The listing builds one solid part. Answer for the finished solid, in the listing's coordinates (mm). A direction names the side the tool comes from. Coordinates: 2 decimals unless noted, no trailing zeros. Write each loop counter-clockwise with the first axis right and the second up, starting at its lowest first coordinate (ties: lowest second). Pieces come first, ordered by that corner, then holes.
(1) For a pull along Z with two mould halves and no side action, classify faces 1 (the cylindrical face through (-1.669, 1.972, -23.347)), 2 (the cylindrical face through (12.61, 1.97, 8.82)), 3 (the cylindrical face through (6.76, 1.97, 10.83)), 4 (the cylindrical face through (6.792, 1.972, 6.686)) as +Z half, -Z half, draft (parallel to the pull), parting line (faces both ways), or undercut.
(2) The part is cut by section A-A on x = -2.5. Determine the outline of the cut face in (y, z), plus the area to 3 significant figures.
(3) The part is cut by section B-B on z = -19.5. Determine the outline of the cut face in (x, y).
(4) The part is cut by section D-D on x = 7. Determine the outline of the cut face in (y, z).
(5) Which of the six approach directions +Z, -Z, +X, -X, +Y, -Y give full straight-line access (tool end or side, diameter ignored) to faces 5 (the flat face through (4.24, 1.97, -0.21)), 6 (the flat face through (-3.874, 1.972, 19.331)), 7 (the cylindrical face through (0.325, 1.972, 17.289)), 8 (the flat face through (7.2, 2, 2.8)), 9 (the flat face through (0, 0, 5))?
(6) Straight lines are drawn through the part: line 1 (Z direction, x = 6.5, y = 2.9); line 2 (Z direction, x = -2.25, y = 3.1); line 3 (X direction, y = 3, z = -6). For each, find the intervals that lie inside material, in ascending order.
(7) Given P1, Ø2, axis at y = 2, z = -13.5, coming from the -X side; P2, Ø1.5, axis at y = 1.5, z = 2, coming from the +X side, each flat-ended and moving along its own axis, determine where each tip first touches the part or whether it passes through.
(8) The part is cut by section C-C on y = 0.75. Give the number of separate pieces and of enclosed holes in the cut face, plus the area to 3 significant figures.
from build123d import *

# Parameters (mm, degrees)
CROQUIS1_R              = 1.500000449
CROQUIS1_R_2            = 1.500000067
SALIENTE_EXTRUIR1_DEPTH = 4


with BuildPart() as part:
    # Croquis1 → Saliente-Extruir1 (new body)
    with BuildSketch(Plane(origin=(0, 0, 0), x_dir=(1, 0, 0), z_dir=(0, 1, 0))):
        with BuildLine():
            Line((7.803034841, -10.666075678), (9.826177161, -11.05442464))
            ThreePointArc((9.826177161, -11.05442464), (12.611497219, -8.758438746), (9.837059372, -6.449314739))
            Line((9.837059372, -6.449314739), (7.783190104, -6.83350636))
            ThreePointArc((7.783190104, -6.83350636), (6.778877321, -6.678958506), (6.091539896, -5.930562574))
            Line((6.091539896, -5.930562574), (5.8088579, -5.271694401))
            ThreePointArc((5.8088579, -5.271694401), (5.746747512, -4.205872048), (6.380859817, -3.346956119))
            Line((6.380859817, -3.346956119), (8.045875641, -2.237519038))
            ThreePointArc((8.045875641, -2.237519038), (8.404769789, 1.386225416), (4.781168268, 1.025891001))
            Line((4.781168268, 1.025891001), (3.675334506, -0.635147383))
            ThreePointArc((3.675334506, -0.635147383), (2.774259756, -1.283481634), (1.669267023, -1.177349334))
            Line((1.669267023, -1.177349334), (1.3673448, -1.048666977))
            Line((1.3673448, -1.048666977), (1.3673448, 20.24263647))
            ThreePointArc((1.3673448, 20.24263647), (-1.737654981, 23.347636251), (-4.842654762, 20.24263647))
            Line((-4.842654762, 20.24263647), (-4.842654762, 0.571999527))
            ThreePointArc((-4.842654762, 0.571999527), (-11.591302814, -9.338185795), (-3.698262021, -18.363479735))
            Line((-3.698262021, -18.363479735), (-4.053895188, -20.326281833))
            ThreePointArc((-4.053895188, -20.326281833), (-1.716098294, -23.09980655), (0.570509604, -20.283930489))
            Line((0.570509604, -20.283930489), (0.177742699, -18.321752082))
            ThreePointArc((0.177742699, -18.321752082), (0.331674177, -17.275555509), (1.114410942, -16.564538403))
            Line((1.114410942, -16.564538403), (1.762991063, -16.295067607))
            ThreePointArc((1.762991063, -16.295067607), (2.82080022, -16.242583246), (3.671047948, -16.874084331))
            Line((3.671047948, -16.874084331), (4.780498307, -18.539119038))
            ThreePointArc((4.780498307, -18.539119038), (8.406487962, -18.895762792), (8.038611241, -15.270895558))
            Line((8.038611241, -15.270895558), (6.389450023, -14.179385265))
            ThreePointArc((6.389450023, -14.179385265), (5.741374186, -13.307833185), (5.800109712, -12.223326174))
            Line((5.800109712, -12.223326174), (6.067644855, -11.592044841))
            ThreePointArc((6.067644855, -11.592044841), (6.771618308, -10.822224208), (7.803034841, -10.666075678))
        make_face()
        with Locations((-1.73765539, 20.242635654)):
            Circle(CROQUIS1_R, mode=Mode.SUBTRACT)
        with Locations((-1.737655616, -8.757364808)):
            Circle(CROQUIS1_R_2, mode=Mode.SUBTRACT)
    extrude(amount=SALIENTE_EXTRUIR1_DEPTH)


solid = part.part
Model answer:
1. face 1: -Z half
1. face 2: parting line
1. face 3: undercut
1. face 4: undercut
2. outline: (0, -23.25) - (4, -23.25) - (4, -21.53) - (0, -21.53) - close; (0, -18.95) - (4, -18.95) - (4, 7.47) - (0, 7.47) - close; (0, 10.05) - (4, 10.05) - (4, 22.97) - (0, 22.97) - close
2. area: 164 mm2
3. outline: (-4.84, 0) - (-3.04, 0) - (-3.04, 4) - (-4.84, 4) - close; (-0.43, 0) - (1.37, 0) - (1.37, 4) - (-0.43, 4) - close
4. outline: (0, -2.06) - (4, -2.06) - (4, 2.93) - (0, 2.93) - close; (0, 6.78) - (4, 6.78) - (4, 10.72) - (0, 10.72) - close; (0, 14.58) - (4, 14.58) - (4, 19.57) - (0, 19.57) - close
5. face 5: -Z, +Y, -Y
5. face 6: -X, +Y, -Y
5. face 7: +Y, -Y
5. face 8: +X, +Y, -Y
5. face 9: +Z, -Z, +X, -X, -Y
6. line 1: z = -2.06 to 3.27, 6.49 to 11.01, 14.25 to 19.58
6. line 2: z = -23.31 to -21.65, -18.83 to 7.35, 10.17 to 23.04
6. line 3: x = -4.84 to 1.37
7. P1: stops at x = -4.84
7. P2: stops at x = 8.88
8. separate pieces: 1
8. enclosed holes: 2
8. area: 482 mm2
